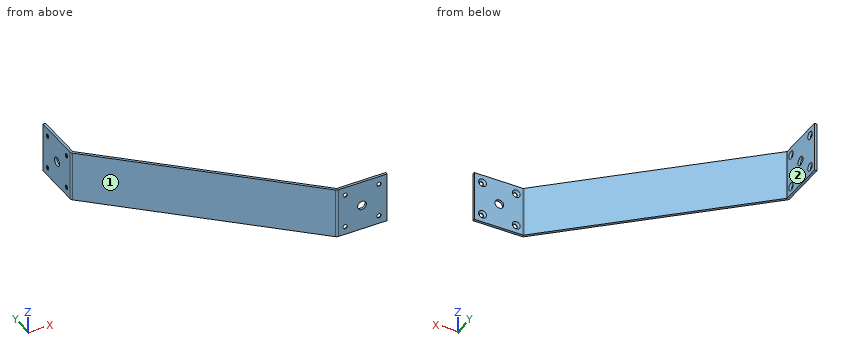
```python
from build123d import *

# Parameters (mm, degrees)
SM_BASE_FLANGE_1_DEPTH              = 40
HOLE_WIZARD_M3_3_AT_2_COUNT         = 2
HOLE_WIZARD_M3_3_AT_2_PITCH         = 27
HOLE_WIZARD_M3_3_AT_3_COUNT         = 2
HOLE_WIZARD_M3_3_AT_3_PITCH         = 38.183766184
HOLE_WIZARD_M3_3_AT_4_COUNT         = 2
HOLE_WIZARD_M3_3_AT_4_PITCH         = 27
HOLE_WIZARD_M3_5_AT_2_COUNT         = 2
HOLE_WIZARD_M3_5_AT_2_PITCH         = 27
HOLE_WIZARD_M3_5_AT_3_COUNT         = 2
HOLE_WIZARD_M3_5_AT_3_PITCH         = 38.183766184
HOLE_WIZARD_M3_5_AT_4_COUNT         = 2
HOLE_WIZARD_M3_5_AT_4_PITCH         = 27
HOLE_WIZARD_7_0_7_1_D               = 7
HOLE_WIZARD_7_0_7_1_DEPTH           = 2
HOLE_WIZARD_7_0_7_1_TIP             = 2.103012167
HOLE_WIZARD_7_0_7_1_ON_FACE_2_D     = 7
HOLE_WIZARD_7_0_7_1_ON_FACE_2_DEPTH = 2
HOLE_WIZARD_7_0_7_1_ON_FACE_2_TIP   = 2.103012167


# Sheet-metal steps are written as plain solids
with BuildPart() as part:
    # Sketch 1 → 基材-凸緣1 (new body)
    with BuildSketch(Plane.XY):
        with BuildLine():
            Line((0, 170), (0, 131.193347828))
            ThreePointArc((0, 131.193347828), (0.228127962, 130.099479649), (0.874477521, 129.187985159))
            Line((0.874477521, 129.187985159), (139.212513644, 0.731237331))
            ThreePointArc((139.212513644, 0.731237331), (140.07436014, 0.189360804), (141.074636122, 0))
            Line((141.074636122, 0), (180, 0))
            Line((180, 0), (180, 2))
            Line((180, 2), (141.074636122, 2))
            ThreePointArc((141.074636122, 2), (140.805395719, 2.050969513), (140.573415842, 2.196824314))
            Line((140.573415842, 2.196824314), (2.23537972, 130.653572142))
            ThreePointArc((2.23537972, 130.653572142), (2.061404318, 130.898915576), (2, 131.193347828))
            Line((2, 131.193347828), (2, 170))
            Line((2, 170), (0, 170))
        make_face()
    extrude(amount=SM_BASE_FLANGE_1_DEPTH)

    # 草圖5 → M3 平錐坑頭螺釘的錐孔3 (revolve, cut)
    with BuildSketch(Plane(origin=(173.5, 2, 6.5), x_dir=(0, 0, 1), z_dir=(1, 0, 0))):
        Polygon((0, 0), (0, 2), (1.7, 2), (1.7, 1.45), (3.15, 0), align=None)
    hole_wizard_m3_3 = revolve(axis=Axis((173.5, 8.35, 6.5), (0, -1, 0)), mode=Mode.SUBTRACT)

    # M3 平錐坑頭螺釘的錐孔3 at 2: M3 平錐坑頭螺釘的錐孔3 ×2
    with Locations(*[(0, 0, i * HOLE_WIZARD_M3_3_AT_2_PITCH) for i in range(1, HOLE_WIZARD_M3_3_AT_2_COUNT)]):
        add(hole_wizard_m3_3, mode=Mode.SUBTRACT)

    # M3 平錐坑頭螺釘的錐孔3 at 3: M3 平錐坑頭螺釘的錐孔3 ×2
    with Locations(*[Vector(-0.7071067811865471, 0, 0.7071067811865479) * (i * HOLE_WIZARD_M3_3_AT_3_PITCH) for i in range(1, HOLE_WIZARD_M3_3_AT_3_COUNT)]):
        add(hole_wizard_m3_3, mode=Mode.SUBTRACT)

    # M3 平錐坑頭螺釘的錐孔3 at 4: M3 平錐坑頭螺釘的錐孔3 ×2
    with Locations(*[(-i * HOLE_WIZARD_M3_3_AT_4_PITCH, 0, 0) for i in range(1, HOLE_WIZARD_M3_3_AT_4_COUNT)]):
        add(hole_wizard_m3_3, mode=Mode.SUBTRACT)

    # 草圖9 → M3 平錐坑頭螺釘的錐孔5 (revolve, cut)
    with BuildSketch(Plane(origin=(2, 163.5, 6.5), x_dir=(0, 0, -1), z_dir=(0, 1, 0))):
        Polygon((0, 0), (0, 2), (1.7, 2), (1.7, 1.45), (3.15, 0), align=None)
    hole_wizard_m3_5 = revolve(axis=Axis((8.35, 163.5, 6.5), (-1, 0, 0)), mode=Mode.SUBTRACT)

    # M3 平錐坑頭螺釘的錐孔5 at 2: M3 平錐坑頭螺釘的錐孔5 ×2
    with Locations(*[(0, -i * HOLE_WIZARD_M3_5_AT_2_PITCH, 0) for i in range(1, HOLE_WIZARD_M3_5_AT_2_COUNT)]):
        add(hole_wizard_m3_5, mode=Mode.SUBTRACT)

    # M3 平錐坑頭螺釘的錐孔5 at 3: M3 平錐坑頭螺釘的錐孔5 ×2
    with Locations(*[Vector(0, -0.7071067811865476, 0.7071067811865476) * (i * HOLE_WIZARD_M3_5_AT_3_PITCH) for i in range(1, HOLE_WIZARD_M3_5_AT_3_COUNT)]):
        add(hole_wizard_m3_5, mode=Mode.SUBTRACT)

    # M3 平錐坑頭螺釘的錐孔5 at 4: M3 平錐坑頭螺釘的錐孔5 ×2
    with Locations(*[(0, 0, i * HOLE_WIZARD_M3_5_AT_4_PITCH) for i in range(1, HOLE_WIZARD_M3_5_AT_4_COUNT)]):
        add(hole_wizard_m3_5, mode=Mode.SUBTRACT)

    # Ø7.0 (7) 直徑孔1
    with Locations(Plane(origin=(2, 150, 20), x_dir=(0, 0, 1), z_dir=(1, 0, 0))):
        with Locations((0, 0)):
            Hole(HOLE_WIZARD_7_0_7_1_D / 2, depth=HOLE_WIZARD_7_0_7_1_DEPTH)
            with Locations((0, 0, -(HOLE_WIZARD_7_0_7_1_DEPTH + HOLE_WIZARD_7_0_7_1_TIP / 2))):  # 118° drill point
                Cone(0, HOLE_WIZARD_7_0_7_1_D / 2, HOLE_WIZARD_7_0_7_1_TIP, mode=Mode.SUBTRACT)

    # Ø7.0 (7) 直徑孔1 on face 2
    with Locations(Plane(origin=(160, 2, 20), x_dir=(0, 0, 1), z_dir=(0, 1, 0))):
        with Locations((0, 0)):
            Hole(HOLE_WIZARD_7_0_7_1_ON_FACE_2_D / 2, depth=HOLE_WIZARD_7_0_7_1_ON_FACE_2_DEPTH)
            with Locations((0, 0, -(HOLE_WIZARD_7_0_7_1_ON_FACE_2_DEPTH + HOLE_WIZARD_7_0_7_1_ON_FACE_2_TIP / 2))):  # 118° drill point
                Cone(0, HOLE_WIZARD_7_0_7_1_ON_FACE_2_D / 2, HOLE_WIZARD_7_0_7_1_ON_FACE_2_TIP, mode=Mode.SUBTRACT)


solid = part.part
```
Model file for the job. Use its own axes, mm. Face numbers are marked on the shaded views. A direction names the side the tool comes from. Coordinates: 2 decimals unless noted, no trailing zeros. Loops run counter-clockwise (first coordinate to the right, second up) from the corner with the lowest first, then second, coordinate; pieces in that order, holes last. Notation, with made-up numbers: (64.25, 1) - (73.25, 1) arc R20 cw to (73.25, 24) - close; hole circle Ø10 at (64, 83.25). An arc over 180 degrees is marked (long way). Write item = value, one per line. Start each with the question number.
Item 1: Saw through at D-D, the plane y = 126. List the corners of the cut face in (x, z).
Item 2: Saw through at B-B, the plane y = 150. List the corners of the cut face in (x, z), then the cut area to 3 significant figures.
Item 3: Saw through at C-C, the plane x = 32. List the corners of the cut face in (y, z) (3 decimals), then the cut area to 3 significant figures.
Item 4: Saw through at A-A, the plane z = 20. List the corners of the cut face in (x, y).
Item 5: 3-axis set-ups, long thin cutter, end or side, ignore diameter. For the marked faces 1 and 2: which of +Z, -Z, +X, -X, +Y, -Y reach the whole face in a straight line?
Item 6: Wall check: probe 1 along Z at (x, y) = (173.5, 0.3); probe 2 along Y at (x, z) = (0.35, 33.5); probe 3 along Z at (x, y) = (1.05, 150). Give the ranges that are in metal, low to high. Write a range as [from, to].
Item 7: Drop flat-ended pins along their axis: pin 1 Ø11 at (y, z) = (150, 20) entering from -X; pin 2 Ø3 at (x, z) = (65, 27.5) entering from -Y; pin 3 Ø3 at (x, z) = (146.5, 6.5) entering from +Y; pin 4 Ø5 at (y, z) = (99, 26) entering from +X. Give the stop position or say it passes through.
Answers:
q1.outline = (4.31, 0) - (7.25, 0) - (7.25, 40) - (4.31, 40) - close
q2.outline = (0, 0) - (2, 0) - (2, 16.5) - (0, 16.5) - close; (0, 23.5) - (2, 23.5) - (2, 40) - (0, 40) - close
q2.area = 66.0 mm2
q3.outline = (100.286, 0) - (103.015, 0) - (103.015, 40) - (100.286, 40) - close
q3.area = 109 mm2
q4.outline = (0, 131.19) arc R2.74 ccw to (0.87, 129.19) - (139.21, 0.73) arc R2.74 ccw to (141.07, 0) - (156.5, 0) - (156.5, 2) - (141.07, 2) arc R0.74 cw to (140.57, 2.2) - (2.24, 130.65) arc R0.74 cw to (2, 131.19) - (2, 146.5) - (0, 146.5) - close; (0, 153.5) - (2, 153.5) - (2, 170) - (0, 170) - close; (163.5, 0) - (180, 0) - (180, 2) - (163.5, 2) - close
q5.face_1 = +Z, -Z, -X, -Y
q5.face_2 = +Z, -Z, +X, +Y
q6.probe_1 = [0, 4.8], [8.2, 31.8], [35.2, 40]
q6.probe_2 = [129.85, 134.8], [138.2, 161.8], [165.2, 170]
q6.probe_3 = [0, 16.5], [23.5, 40]
q7.pin_1 = 0
q7.pin_2 = 68.25
q7.pin_3 = through
q7.pin_4 = 39.02
